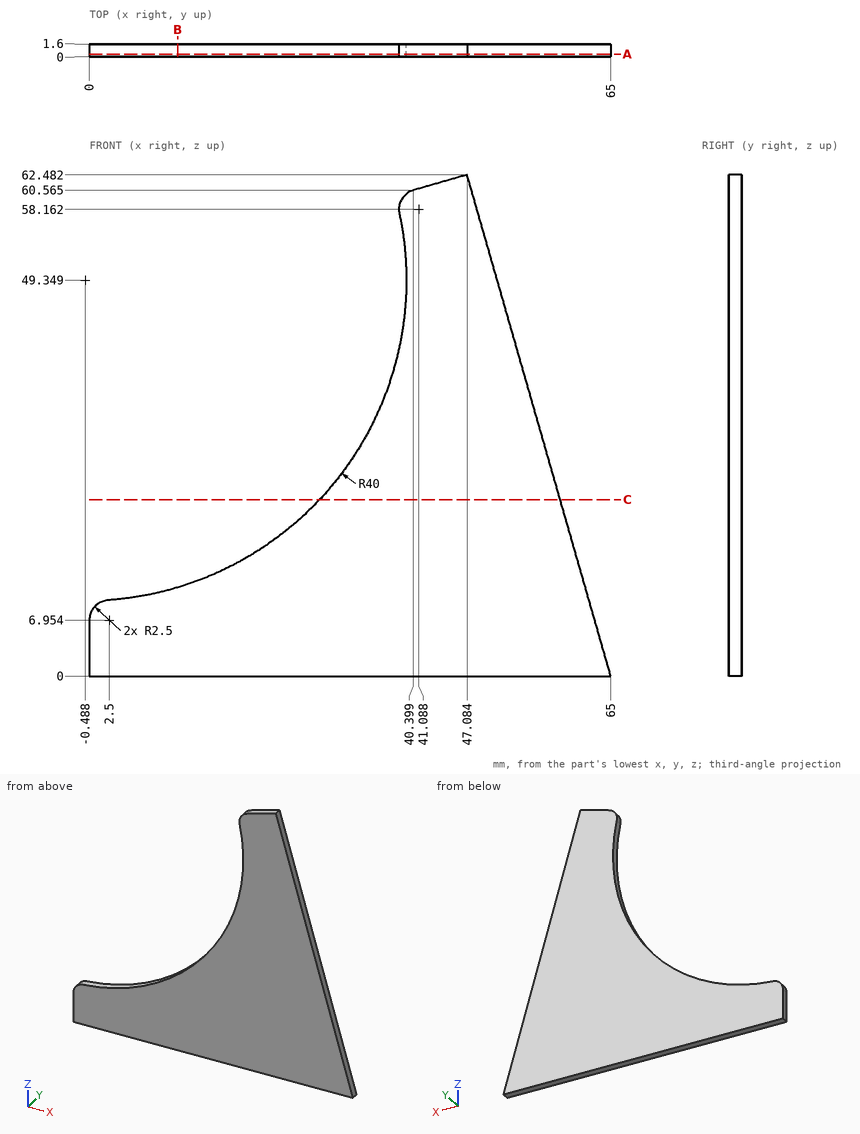
Design review of the part shown in the three views and the two pictorial views. Dimensions are in mm from the part's minimum x, y and z. Coordinates: 2 decimals unless noted, no trailing zeros. Order: outer loops, then holes, each group sorted by start corner. A loop starts at its lowest first (then second) coordinate and runs counter-clockwise, first axis right, second up. Notation, with made-up numbers: (35.5, 33) - (74.5, 33) arc R14 cw to (74.5, 50) - close; hole circle Ø11 at (16.5, -10). An arc over 180 degrees is marked (long way). Answer as CSV lines item,"result". Start each with the question number.
1) Add section B-B (x = 11). State the section outline as (y, z) points.
2) Add section A-A (y = 0.35). State the section outline as (x, z) points (1 decimal).
3) Add section C-C (z = 22). State the section outline as (x, y) points.
4) Insertion check: P1, Ø12, axis at x = 13, z = 18.5, coming from the -Y side. The pin has a flat end and moves straight along its axis. Give the tip position at first contact, or say it passes through.
5) To check wall thickness, follow line 1 along X through (y, z) = (0.4, 36.5) (1 decimal); line 2 along Z through (x, y) = (30, 1.4) (1 decimal); line 3 along X through (y, z) = (1.15, 37.5). State the ranges of each line that lie inside material, in increasing order. Write a range as [from, to].
Result:
1,outline,"(0, 0) - (1.6, 0) - (1.6, 11.03) - (0, 11.03) - close"
2,outline,"(0, 0) - (65, 0) - (47.1, 62.5) - (40.4, 60.6) arc R2.5 ccw to (38.6, 57.6) arc R40 cw to (2.3, 9.4) arc R2.5 ccw to (0, 7) - close"
3,outline,"(28.7, 0) - (58.69, 0) - (58.69, 1.6) - (28.7, 1.6) - close"
4,P1,"through"
5,line 1,"[37.4, 54.5]"
5,line 2,"[0, 23.5]"
5,line 3,"[37.72, 54.25]"
